Here's how the part is built. I have some questions about the finished solid (model axes, mm). Give positions to 0.01 mm unless a question says otherwise; leave off trailing zeros. Write each loop counter-clockwise with the first axis right and the second up, starting at its lowest first coordinate (ties: lowest second). Pieces come first, ordered by that corner, then holes. Notation, with made-up numbers: (-18.75, -31.5) - (-8.75, -31.5) arc R20 cw to (-8.75, -22.5) - close; hole circle Ø10 at (40, -17.5). An arc over 180 degrees is marked (long way). Use a Markdown table: item, result.
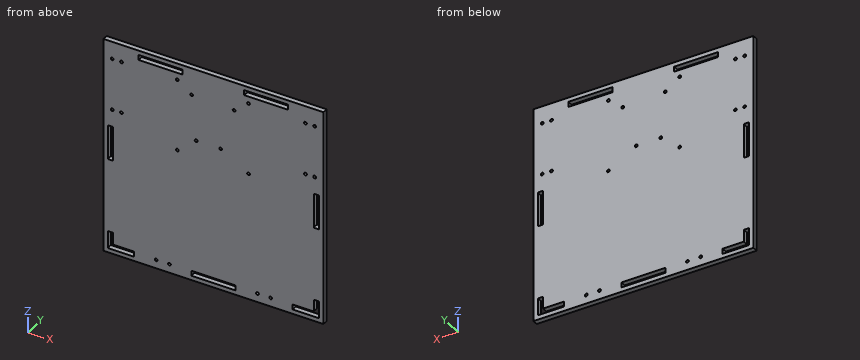
```python
from build123d import *

# Parameters (mm, degrees)
SKETCH1_W           = 250
SKETCH1_H           = 250
BOSS_EXTRUDE1_DEPTH = 6
CUT_EXTRUDE2_REACH  = 8
SKETCH4_R           = 1.6
CUT_EXTRUDE3_REACH  = 8
SKETCH5_R           = 1.6
SKETCH6_W           = 6
SKETCH6_H           = 40
SKETCH6_W_2         = 50
SKETCH6_H_2         = 6
CUT_EXTRUDE6_DEPTH  = 6
CUT_EXTRUDE7_REACH  = 8
SKETCH7_R           = 1.6
CUT_EXTRUDE8_REACH  = 8
SKETCH8_R           = 1.6


with BuildPart() as part:
    # Sketch1 → Boss-Extrude1 (new body)
    with BuildSketch(Plane(origin=(0, 0, 0), x_dir=(1, 0, 0), z_dir=(0, 1, 0))):
        Rectangle(SKETCH1_W, SKETCH1_H)
    extrude(amount=BOSS_EXTRUDE1_DEPTH)

    # Sketch4 → Cut-Extrude2 (cut, up to next)
    with BuildSketch(Plane(origin=(0, 6, 0), x_dir=(1, 0, 0), z_dir=(0, 1, 0)), mode=Mode.PRIVATE) as cut_extrude2_sk1:
        with Locations((-115, -105)):
            Circle(SKETCH4_R)
    cut_extrude2_tool1 = extrude(cut_extrude2_sk1.sketch, amount=-CUT_EXTRUDE2_REACH, mode=Mode.PRIVATE) & part.part
    add(cut_extrude2_tool1.solids().sort_by_distance((-115, 6, 105))[0], mode=Mode.SUBTRACT)
    # Sketch4 → Cut-Extrude2 (cut, up to next)
    with BuildSketch(Plane(origin=(0, 6, 0), x_dir=(1, 0, 0), z_dir=(0, 1, 0)), mode=Mode.PRIVATE) as cut_extrude2_sk2:
        with Locations((-104.5, -105)):
            Circle(SKETCH4_R)
    cut_extrude2_tool2 = extrude(cut_extrude2_sk2.sketch, amount=-CUT_EXTRUDE2_REACH, mode=Mode.PRIVATE) & part.part
    add(cut_extrude2_tool2.solids().sort_by_distance((-104.5, 6, 105))[0], mode=Mode.SUBTRACT)
    # Sketch4 → Cut-Extrude2 (cut, up to next)
    with BuildSketch(Plane(origin=(0, 6, 0), x_dir=(1, 0, 0), z_dir=(0, 1, 0)), mode=Mode.PRIVATE) as cut_extrude2_sk3:
        with Locations((-115, -45)):
            Circle(SKETCH4_R)
    cut_extrude2_tool3 = extrude(cut_extrude2_sk3.sketch, amount=-CUT_EXTRUDE2_REACH, mode=Mode.PRIVATE) & part.part
    add(cut_extrude2_tool3.solids().sort_by_distance((-115, 6, 45))[0], mode=Mode.SUBTRACT)
    # Sketch4 → Cut-Extrude2 (cut, up to next)
    with BuildSketch(Plane(origin=(0, 6, 0), x_dir=(1, 0, 0), z_dir=(0, 1, 0)), mode=Mode.PRIVATE) as cut_extrude2_sk4:
        with Locations((-104.5, -45)):
            Circle(SKETCH4_R)
    cut_extrude2_tool4 = extrude(cut_extrude2_sk4.sketch, amount=-CUT_EXTRUDE2_REACH, mode=Mode.PRIVATE) & part.part
    add(cut_extrude2_tool4.solids().sort_by_distance((-104.5, 6, 45))[0], mode=Mode.SUBTRACT)
    # Sketch4 → Cut-Extrude2 (cut, up to next)
    with BuildSketch(Plane(origin=(0, 6, 0), x_dir=(1, 0, 0), z_dir=(0, 1, 0)), mode=Mode.PRIVATE) as cut_extrude2_sk5:
        with Locations((115, -45)):
            Circle(SKETCH4_R)
    cut_extrude2_tool5 = extrude(cut_extrude2_sk5.sketch, amount=-CUT_EXTRUDE2_REACH, mode=Mode.PRIVATE) & part.part
    add(cut_extrude2_tool5.solids().sort_by_distance((115, 6, 45))[0], mode=Mode.SUBTRACT)
    # Sketch4 → Cut-Extrude2 (cut, up to next)
    with BuildSketch(Plane(origin=(0, 6, 0), x_dir=(1, 0, 0), z_dir=(0, 1, 0)), mode=Mode.PRIVATE) as cut_extrude2_sk6:
        with Locations((104.5, -45)):
            Circle(SKETCH4_R)
    cut_extrude2_tool6 = extrude(cut_extrude2_sk6.sketch, amount=-CUT_EXTRUDE2_REACH, mode=Mode.PRIVATE) & part.part
    add(cut_extrude2_tool6.solids().sort_by_distance((104.5, 6, 45))[0], mode=Mode.SUBTRACT)
    # Sketch4 → Cut-Extrude2 (cut, up to next)
    with BuildSketch(Plane(origin=(0, 6, 0), x_dir=(1, 0, 0), z_dir=(0, 1, 0)), mode=Mode.PRIVATE) as cut_extrude2_sk7:
        with Locations((115, -105)):
            Circle(SKETCH4_R)
    cut_extrude2_tool7 = extrude(cut_extrude2_sk7.sketch, amount=-CUT_EXTRUDE2_REACH, mode=Mode.PRIVATE) & part.part
    add(cut_extrude2_tool7.solids().sort_by_distance((115, 6, 105))[0], mode=Mode.SUBTRACT)
    # Sketch4 → Cut-Extrude2 (cut, up to next)
    with BuildSketch(Plane(origin=(0, 6, 0), x_dir=(1, 0, 0), z_dir=(0, 1, 0)), mode=Mode.PRIVATE) as cut_extrude2_sk8:
        with Locations((104.5, -105)):
            Circle(SKETCH4_R)
    cut_extrude2_tool8 = extrude(cut_extrude2_sk8.sketch, amount=-CUT_EXTRUDE2_REACH, mode=Mode.PRIVATE) & part.part
    add(cut_extrude2_tool8.solids().sort_by_distance((104.5, 6, 105))[0], mode=Mode.SUBTRACT)

    # Sketch5 → Cut-Extrude3 (cut, up to next)
    with BuildSketch(Plane(origin=(0, 6, 0), x_dir=(1, 0, 0), z_dir=(0, 1, 0)), mode=Mode.PRIVATE) as cut_extrude3_sk1:
        with Locations((-65, 115)):
            Circle(SKETCH5_R)
    cut_extrude3_tool1 = extrude(cut_extrude3_sk1.sketch, amount=-CUT_EXTRUDE3_REACH, mode=Mode.PRIVATE) & part.part
    add(cut_extrude3_tool1.solids().sort_by_distance((-65, 6, -115))[0], mode=Mode.SUBTRACT)
    # Sketch5 → Cut-Extrude3 (cut, up to next)
    with BuildSketch(Plane(origin=(0, 6, 0), x_dir=(1, 0, 0), z_dir=(0, 1, 0)), mode=Mode.PRIVATE) as cut_extrude3_sk2:
        with Locations((-50, 115)):
            Circle(SKETCH5_R)
    cut_extrude3_tool2 = extrude(cut_extrude3_sk2.sketch, amount=-CUT_EXTRUDE3_REACH, mode=Mode.PRIVATE) & part.part
    add(cut_extrude3_tool2.solids().sort_by_distance((-50, 6, -115))[0], mode=Mode.SUBTRACT)
    # Sketch5 → Cut-Extrude3 (cut, up to next)
    with BuildSketch(Plane(origin=(0, 6, 0), x_dir=(1, 0, 0), z_dir=(0, 1, 0)), mode=Mode.PRIVATE) as cut_extrude3_sk3:
        with Locations((50, 115)):
            Circle(SKETCH5_R)
    cut_extrude3_tool3 = extrude(cut_extrude3_sk3.sketch, amount=-CUT_EXTRUDE3_REACH, mode=Mode.PRIVATE) & part.part
    add(cut_extrude3_tool3.solids().sort_by_distance((50, 6, -115))[0], mode=Mode.SUBTRACT)
    # Sketch5 → Cut-Extrude3 (cut, up to next)
    with BuildSketch(Plane(origin=(0, 6, 0), x_dir=(1, 0, 0), z_dir=(0, 1, 0)), mode=Mode.PRIVATE) as cut_extrude3_sk4:
        with Locations((65, 115)):
            Circle(SKETCH5_R)
    cut_extrude3_tool4 = extrude(cut_extrude3_sk4.sketch, amount=-CUT_EXTRUDE3_REACH, mode=Mode.PRIVATE) & part.part
    add(cut_extrude3_tool4.solids().sort_by_distance((65, 6, -115))[0], mode=Mode.SUBTRACT)

    # Sketch6 → Cut-Extrude6 (cut)
    with BuildSketch(Plane(origin=(0, 6, 0), x_dir=(1, 0, 0), z_dir=(0, 1, 0))):
        Polygon((-90, 120), (-120, 120), (-120, 100), (-114, 100), (-114, 114), (-90, 114), align=None)
        with Locations((-117, -5)):
            Rectangle(SKETCH6_W, SKETCH6_H)
        with Locations((-60, -117)):
            Rectangle(SKETCH6_W_2, SKETCH6_H_2)
        with Locations((60, -117)):
            Rectangle(SKETCH6_W_2, SKETCH6_H_2)
        Polygon((120, 100), (120, 120), (90, 120), (90, 114), (114, 114), (114, 100), align=None)
        with Locations((117, -5)):
            Rectangle(SKETCH6_W, SKETCH6_H)
        with Locations((0, 117)):
            Rectangle(SKETCH6_W_2, SKETCH6_H_2)
    extrude(amount=-CUT_EXTRUDE6_DEPTH, mode=Mode.SUBTRACT)

    # Sketch7 → Cut-Extrude7 (cut, up to next)
    with BuildSketch(Plane(origin=(0, 0, 0), x_dir=(-1, 0, 0), z_dir=(0, -1, 0)), mode=Mode.PRIVATE) as cut_extrude7_sk1:
        with Locations((19.693028717, -41.4)):
            Circle(SKETCH7_R)
    cut_extrude7_tool1 = extrude(cut_extrude7_sk1.sketch, amount=-CUT_EXTRUDE7_REACH, mode=Mode.PRIVATE) & part.part
    add(cut_extrude7_tool1.solids().sort_by_distance((-19.693029, 0, 41.4))[0], mode=Mode.SUBTRACT)
    # Sketch7 → Cut-Extrude7 (cut, up to next)
    with BuildSketch(Plane(origin=(0, 0, 0), x_dir=(-1, 0, 0), z_dir=(0, -1, 0)), mode=Mode.PRIVATE) as cut_extrude7_sk2:
        with Locations((-8.206971283, -41.4)):
            Circle(SKETCH7_R)
    cut_extrude7_tool2 = extrude(cut_extrude7_sk2.sketch, amount=-CUT_EXTRUDE7_REACH, mode=Mode.PRIVATE) & part.part
    add(cut_extrude7_tool2.solids().sort_by_distance((8.206971, 0, 41.4))[0], mode=Mode.SUBTRACT)
    # Sketch7 → Cut-Extrude7 (cut, up to next)
    with BuildSketch(Plane(origin=(0, 0, 0), x_dir=(-1, 0, 0), z_dir=(0, -1, 0)), mode=Mode.PRIVATE) as cut_extrude7_sk3:
        with Locations((-23.506971283, -92.2)):
            Circle(SKETCH7_R)
    cut_extrude7_tool3 = extrude(cut_extrude7_sk3.sketch, amount=-CUT_EXTRUDE7_REACH, mode=Mode.PRIVATE) & part.part
    add(cut_extrude7_tool3.solids().sort_by_distance((23.506971, 0, 92.2))[0], mode=Mode.SUBTRACT)
    # Sketch7 → Cut-Extrude7 (cut, up to next)
    with BuildSketch(Plane(origin=(0, 0, 0), x_dir=(-1, 0, 0), z_dir=(0, -1, 0)), mode=Mode.PRIVATE) as cut_extrude7_sk4:
        with Locations((24.793028717, -93.8)):
            Circle(SKETCH7_R)
    cut_extrude7_tool4 = extrude(cut_extrude7_sk4.sketch, amount=-CUT_EXTRUDE7_REACH, mode=Mode.PRIVATE) & part.part
    add(cut_extrude7_tool4.solids().sort_by_distance((-24.793029, 0, 93.8))[0], mode=Mode.SUBTRACT)

    # Sketch8 → Cut-Extrude8 (cut, up to next)
    with BuildSketch(Plane(origin=(0, 0, 0), x_dir=(-1, 0, 0), z_dir=(0, -1, 0)), mode=Mode.PRIVATE) as cut_extrude8_sk1:
        with Locations((41.143028717, -105.838250208)):
            Circle(SKETCH8_R)
    cut_extrude8_tool1 = extrude(cut_extrude8_sk1.sketch, amount=-CUT_EXTRUDE8_REACH, mode=Mode.PRIVATE) & part.part
    add(cut_extrude8_tool1.solids().sort_by_distance((-41.143029, 0, 105.83825))[0], mode=Mode.SUBTRACT)
    # Sketch8 → Cut-Extrude8 (cut, up to next)
    with BuildSketch(Plane(origin=(0, 0, 0), x_dir=(-1, 0, 0), z_dir=(0, -1, 0)), mode=Mode.PRIVATE) as cut_extrude8_sk2:
        with Locations((41.143028717, -22.838250208)):
            Circle(SKETCH8_R)
    cut_extrude8_tool2 = extrude(cut_extrude8_sk2.sketch, amount=-CUT_EXTRUDE8_REACH, mode=Mode.PRIVATE) & part.part
    add(cut_extrude8_tool2.solids().sort_by_distance((-41.143029, 0, 22.83825))[0], mode=Mode.SUBTRACT)
    # Sketch8 → Cut-Extrude8 (cut, up to next)
    with BuildSketch(Plane(origin=(0, 0, 0), x_dir=(-1, 0, 0), z_dir=(0, -1, 0)), mode=Mode.PRIVATE) as cut_extrude8_sk3:
        with Locations((-39.856971283, -22.838250208)):
            Circle(SKETCH8_R)
    cut_extrude8_tool3 = extrude(cut_extrude8_sk3.sketch, amount=-CUT_EXTRUDE8_REACH, mode=Mode.PRIVATE) & part.part
    add(cut_extrude8_tool3.solids().sort_by_distance((39.856971, 0, 22.83825))[0], mode=Mode.SUBTRACT)
    # Sketch8 → Cut-Extrude8 (cut, up to next)
    with BuildSketch(Plane(origin=(0, 0, 0), x_dir=(-1, 0, 0), z_dir=(0, -1, 0)), mode=Mode.PRIVATE) as cut_extrude8_sk4:
        with Locations((-39.856971283, -105.838250208)):
            Circle(SKETCH8_R)
    cut_extrude8_tool4 = extrude(cut_extrude8_sk4.sketch, amount=-CUT_EXTRUDE8_REACH, mode=Mode.PRIVATE) & part.part
    add(cut_extrude8_tool4.solids().sort_by_distance((39.856971, 0, 105.83825))[0], mode=Mode.SUBTRACT)


solid = part.part
```
Item 1: If we section it at B-B, the plane y = 2.85: Count the separate pieces of the cut face and the enclosed holes in it, plus the area to 3 significant figures.
Values:
| item | result |
|---|---|
| separate pieces | 1 |
| enclosed holes | 27 |
| area | 60,400 mm2 |
Item 2: I need wall thicknesses on line 1 along X through (y, z) = (3.4, 41.4); line 2 along Z through (x, y) = (-104.5, 3.5); line 3 along X through (y, z) = (4.75, 14.5). Which ranges of each line are inside material? Lowest first, please. Write a range as [from, to].
Values:
| item | result |
|---|---|
| line 1 | x = [-125, -21.29], [-18.09, 6.61], [9.81, 125] |
| line 2 | z = [-125, -120], [-114, 43.4], [46.6, 103.4], [106.6, 125] |
| line 3 | x = [-125, -120], [-114, 114], [120, 125] |
Item 3: If we section it at A-A, the plane x = -12.5: Write out the boundary of the cut face in (y, z).
Values:
| item | result |
|---|---|
| outline | (0, -125) - (6, -125) - (6, -120) - (0, -120) - close; (0, -114) - (6, -114) - (6, 125) - (0, 125) - close |
